Model file for the job. Use its own axes, mm. Face numbers are marked on the shaded views. Give positions to 0.01 mm unless a question says otherwise; leave off trailing zeros. Order: outer loops, then holes, each group sorted by start corner. A loop starts at its lowest first (then second) coordinate and runs counter-clockwise, first axis right, second up. Notation, with made-up numbers: M -31.5,-2.75 L -9.5,-2.75 A21 cw -9.5,34.25 Z; hole C 75,44 d5. An arc over 180 degrees is marked long. Return JSON: item names as keys, results as strings. Group by question number.
1. Wall check: probe 1 along Y at (x, z) = (0, 66); probe 2 along Z at (x, y) = (-11, -26); probe 3 along Y at (x, z) = (14, 11). Give the ranges that are in metal, low to high. Write a range as [from, to].
2. Slice it at A-A on x = 0. List the corners of the cut face in (y, z), then the cut area to 3 significant figures.
3. Pin check, flat tips, straight feed: pin 1 (6 mm diameter, centred on x = 28.5, z = 73.5, fed in from -Y); pin 2 (2 mm diameter, centred on y = -7, z = 41, fed in from +X); pin 3 (4 mm diameter, centred on y = 14.5, z = 17, fed in from +X). Stop position of each tip, or through.
4. Slice it at C-C on z = 12. List the corners of the cut face in (x, y), then the cut area to 3 significant figures.
5. Two-plate mould, pull along X, no slides. Class the marked faces 1, 2 and 3: released by +X, released by -X, zero draft, split by the parting line, or undercut.
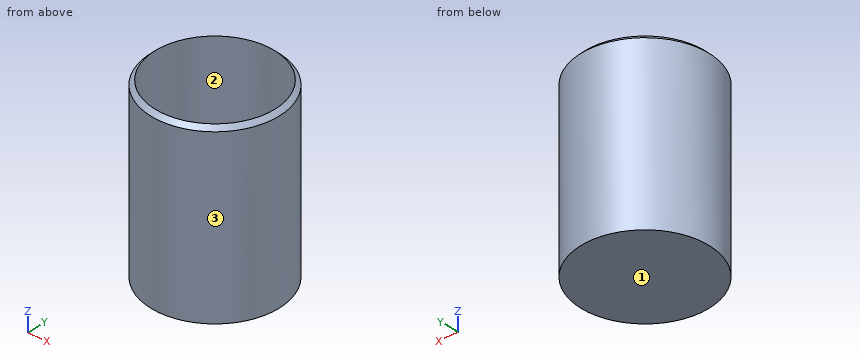
from build123d import *

# Parameters (mm, degrees)
F0_R     = 37.5
F1_DEPTH = 105
F2_R     = 35
F3_DEPTH = 100


# Not quite as in the source:
# - a fillet or chamfer that OpenCascade refuses, or shapes differently, is made with other operations: its cross-section is extruded or revolved along the edge and cut away or added


with BuildPart() as f1:
    # F0 (on Top) → F1 (new body)
    with BuildSketch(Plane.XY):
        Circle(F0_R)
    extrude(amount=F1_DEPTH)

    # F2 (on face) → F3 (cut)
    with BuildSketch(Plane.XY.offset(105)):
        Circle(F2_R)
    extrude(amount=-F3_DEPTH, mode=Mode.SUBTRACT)

    # F4: chamfer of 5 on 1 edges, made by hand

    # F4_s1 → F4_t2 (revolve, cut)
    with BuildSketch(Plane.XZ):
        Polygon((37.5, 100), (32.5, 105), (37.5, 105), align=None)
    revolve(axis=Axis((0, 0, 105), (0, 0, 1)), mode=Mode.SUBTRACT)


solid = f1.part
Result:
{
 "1": {"probe 1": "y = [-37.5, -35], [35, 37.5]", "probe 2": "z = [0, 5]", "probe 3": "y = [-34.79, -32.08], [32.08, 34.79]"},
 "2": {"outline": "M -37.5,0 L 37.5,0 L 37.5,100 L 35,102.5 L 35,5 L -35,5 L -35,102.5 L -37.5,100 Z", "area": "856 mm2"},
 "3": {"pin 1": "stops at y = -27.5", "pin 2": "stops at x = 37.02", "pin 3": "stops at x = 35.36"},
 "4": {"outline": "C 0,0 d75; hole C 0,0 d70", "area": "569 mm2"},
 "5": {"face 1": "zero draft", "face 2": "undercut", "face 3": "split by the parting line"}
}
